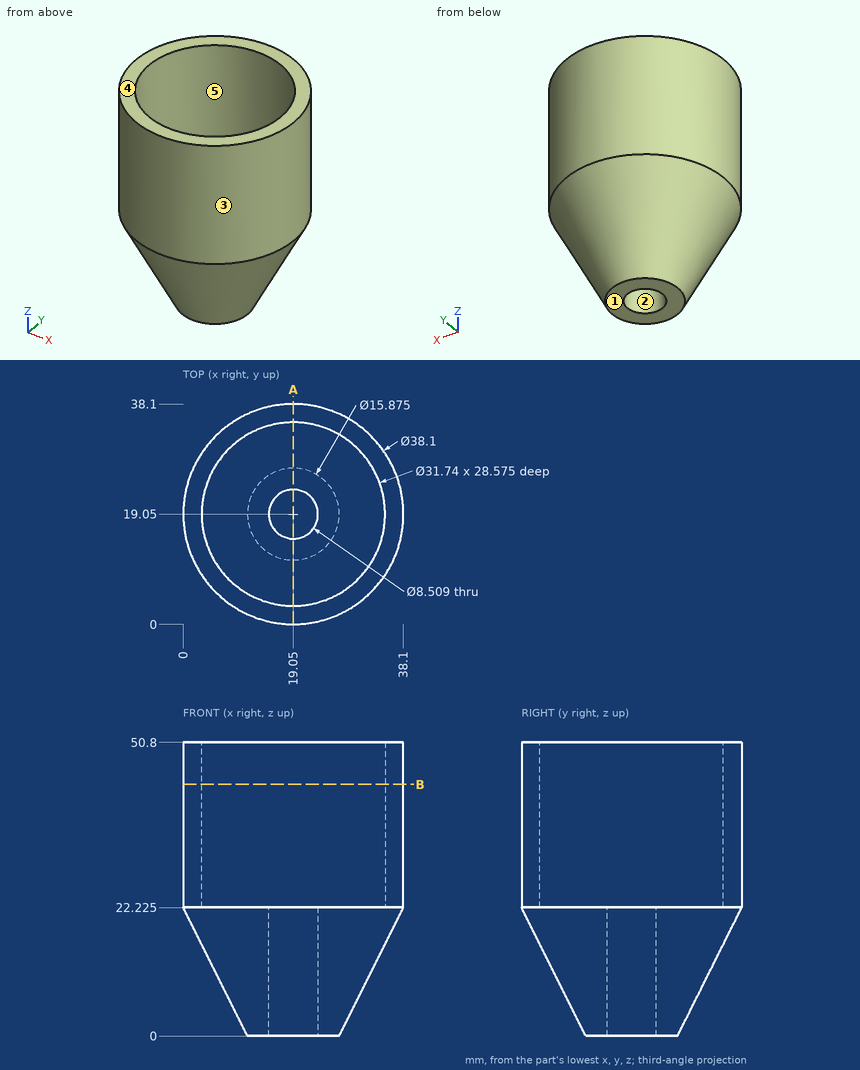
Part print with two shaded views. Sizes in mm from the minimum x, y, z corner. A direction names the side the tool comes from. Coordinates: 2 decimals unless noted, no trailing zeros. Loops run counter-clockwise (first coordinate to the right, second up) from the corner with the lowest first, then second, coordinate; pieces in that order, holes last. Notation, with made-up numbers: (-35.5, 79.5) - (-27.5, 79.5) arc R22 ccw to (-27.5, 102.5) - close; hole circle Ø4 at (80.5, -12). An arc over 180 degrees is marked (long way). Write each question's results on one line, items separated by ' | '. Start each with the question number.
Q1. Slice it at A-A on x = 19.05. Give the cut face in (y, z) (1 decimal).
Q2. Slice it at B-B on z = 43.5. Give the cut face in (x, y), and give its area (3 significant figures).
Q3. Drop flat-ended pins along their axis: pin 1 Ø6 at (x, y) = (11.5, 9) entering from +Z (3 decimals); pin 2 Ø6 at (y, z) = (19, 7.5) entering from -X; pin 3 Ø5 at (y, z) = (8.5, 27) entering from +X (1 decimal). Give the stop position or say it passes through.
Q4. Two-plate mould, pull along Y, no slides. Class the marked faces 1, 2 and 3: +Y half, -Y half, draft (parallel to the pull), parting line (faces both ways), or undercut.
Q5. Probe line 1 along X through (y, z) = (19, 33); line 2 along Y through (x, z) = (23.5, 30); line 3 along X through (y, z) = (19, 5) (1 decimal). List the from-to ranges inside material, lowest first.
Q6. Which spindle directions (+Z, -Z, +X, -X, +Y, -Y) get a long thin tool onto all of the face, cutting with end or side? Do the marked faces 4 and 5. Say none if no direction does.
Answer:
1) outline: (0, 22.2) - (11.1, 0) - (14.8, 0) - (14.8, 22.2) - (3.2, 22.2) - (3.2, 50.8) - (0, 50.8) - close; (23.3, 0) - (27, 0) - (38.1, 22.2) - (38.1, 50.8) - (34.9, 50.8) - (34.9, 22.2) - (23.3, 22.2) - close
2) outline: circle Ø38.1 at (19.05, 19.05); hole circle Ø31.74 at (19.05, 19.05) | area: 349 mm2
3) pin 1: stops at z = 22.225 | pin 2: stops at x = 5.86 | pin 3: stops at x = 36.3
4) face 1: draft | face 2: undercut | face 3: parting line
5) line 1: x = 0 to 3.18, 34.92 to 38.1 | line 2: y = 0.53 to 3.82, 34.28 to 37.57 | line 3: x = 8.6 to 14.8, 23.3 to 29.5
6) face 4: +Z, +X, -X, +Y, -Y | face 5: +Z
